from build123d import *

# Parameters (mm, degrees)
SKETCH1_W                = 38
SKETCH1_H                = 33
SKETCH1_R                = 1.7
BOSS_EXTRUDE1_DEPTH      = 3
BOSS_EXTRUDE2_DEPTH      = 5
BOSS_EXTRUDE2_DEPTH_BACK = 4
SKETCH3_R                = 0.75
SKETCH3_W                = 23.2
SKETCH3_H                = 12.2
FILLET1_R                = 2
CHAMFER1_SIZE            = 1.5
CHAMFER2_SIZE            = 3
CHAMFER2_SIZE_2          = 7


with BuildPart() as part:
    # Sketch1 → Boss-Extrude1 (new body)
    with BuildSketch(Plane.XY):
        Rectangle(SKETCH1_W, SKETCH1_H)
        with Locations((-13, 10.5)):
            Circle(SKETCH1_R, mode=Mode.SUBTRACT)
        with Locations((13, 10.5)):
            Circle(SKETCH1_R, mode=Mode.SUBTRACT)
        with Locations((13, -10.5)):
            Circle(SKETCH1_R, mode=Mode.SUBTRACT)
        with Locations((-13, -10.5)):
            Circle(SKETCH1_R, mode=Mode.SUBTRACT)
    extrude(amount=BOSS_EXTRUDE1_DEPTH)

    # Sketch3 → Boss-Extrude2 (add, two sides: drawn at the far end of the back side and taken through both)
    with BuildSketch(Plane(origin=(0, 0, 0), x_dir=(-1, 0, 0), z_dir=(0, -1, 0)).offset(-BOSS_EXTRUDE2_DEPTH_BACK)):
        Polygon((16.6, -3), (16.6, -16), (12.612805852, -20), (-12.612805852, -20), (-16.6, -16), (-16.6, -3), align=None)
        with Locations(Location((-13.85, -11.6, 0), (0, 0, 90))):
            Circle(SKETCH3_R, mode=Mode.SUBTRACT)
        with Locations(Location((13.85, -11.6, 0), (0, 0, 90))):
            Circle(SKETCH3_R, mode=Mode.SUBTRACT)
        with Locations((0, -11.6)):
            Rectangle(SKETCH3_W, SKETCH3_H, mode=Mode.SUBTRACT)
    extrude(amount=BOSS_EXTRUDE2_DEPTH + BOSS_EXTRUDE2_DEPTH_BACK)

    # Fillet1
    fillet1_edges = [part.edges().sort_by_distance(p)[0] for p in [
        (19, -16.5, 1.5),
        (-19, -16.5, 1.5),
        (-19, 16.5, 1.5),
        (19, 16.5, 1.5),
    ]]
    fillet(fillet1_edges, radius=FILLET1_R)

    # Chamfer1
    chamfer1_edges = [part.edges().sort_by_distance(p)[0] for p in [
        (-14.7, 10.5, 3),
        (11.3, 10.5, 3),
        (11.3, -10.5, 3),
        (-14.7, -10.5, 3),
    ]]
    chamfer(chamfer1_edges, length=CHAMFER1_SIZE)

    # Chamfer2
    # the kernel refuses this chamfer: 7, 3 mm, written as the material it takes off along each edge
    with BuildSketch(Plane(origin=(-11.6, -5, 17.7), x_dir=(-0.9965941369752023, -0.08246287738523173, 0), z_dir=(0, 0, -1))) as chamfer2_piece_1:
        Polygon((CHAMFER2_SIZE * 0.996594136975, CHAMFER2_SIZE * 0.0824628773852), (-CHAMFER2_SIZE_2 * 0.0824628773852, CHAMFER2_SIZE_2 * 0.996594136975), (0, 0), align=None)
    extrude(amount=12.2, mode=Mode.SUBTRACT)


solid = part.part
Part model, mm, in its own coordinate system. A direction names the side the tool comes from. Round coordinates to 2 decimals unless told otherwise and drop trailing zeros. Write each loop counter-clockwise with the first axis right and the second up, starting at its lowest first coordinate (ties: lowest second). Pieces come first, ordered by that corner, then holes. Notation, with made-up numbers: M 24,88.5 L 51,88.5 A25 cw 51,119.5 Z; hole C 43.5,-35 d9. An arc over 180 degrees is marked long. Return JSON: item names as keys, results as strings. Group by question number.
(1) Saw through at D-D on y = -2. Write the cut outline in (x, z), then the cut area to 3 significant figures.
(2) Saw through at B-B on z = 8.5. Write the cut outline in (x, y).
(3) Saw through at A-A on x = -1.5. Write the cut outline in (y, z).
(4) Which spindle directions (+Z, -Z, +X, -X, +Y, -Y) get a long thin tool onto all of the face, cutting with end or side? Do faces 1 (the face through (11.6, 0, 12)), 2 (the face through (2, -5, 5)), 3 (the face through (0, 0, 20)). Say none if no direction does.
(5) Drill centre lines: probe 1 along Y at (x, z) = (-13, 0.8); probe 2 along Z at (x, y) = (-5.5, 0.5); probe 3 along Y at (x, z) = (-12.5, 4.75). Where is each one in solid material? Low to high.
(6) Saw through at C-C on y = -10.5. Write the cut outline in (x, z), then the cut area to 3 significant figures.
(7) Pin check, flat tips, straight feed: pin 1 Ø0.6 at (y, z) = (3.5, 9.5) entering from +X; pin 2 Ø7 at (y, z) = (1, 11.5) entering from -X; pin 3 Ø2.5 at (x, y) = (13, 10.5) entering from +Z; pin 4 Ø6 at (x, y) = (-4, -12.5) entering from +Z. Stop position of each tip, or through.
(8) Two-plate mould, pull along X, no slides. Class faces 4 (the face through (0, 0, 0)), 5 (the face through (-11.6, 3, 12)), 6 (the face through (-19, 0, 1)): +X half, -X half, draft (parallel to the pull), parting line (faces both ways), or undercut.
Returned:
{
 "1": {"outline": "M -19,0 L 19,0 L 19,3 L 16.6,3 L 16.6,16 L 12.61,20 L -12.61,20 L -16.6,16 L -16.6,3 L -19,3 Z; hole M -13.31,5.5 L 11.6,5.5 L 11.6,17.7 L -13.31,17.7 L -13.31,12.12 A0.75 ccw long -13.31,11.08 Z; hole C 13.85,11.6 d1.5", "area": "355 mm²"},
 "2": {"outline": "M -16.6,-5 L -14.6,-5 L -11.6,2 L -11.6,4 L -16.6,4 Z; M 11.6,-5 L 16.6,-5 L 16.6,4 L 11.6,4 Z"},
 "3": {"outline": "M -16.5,0 L 16.5,0 L 16.5,3 L 4,3 L 4,5.5 L -5,5.5 L -5,3 L -16.5,3 Z; M -5,17.7 L 4,17.7 L 4,20 L -5,20 Z"},
 "4": {"face 1": "+Y, -Y", "face 2": "+Z, +X, -X, -Y", "face 3": "+Z, +X, -X, +Y, -Y"},
 "5": {"probe 1": "-16.5 to -12.2, -8.8 to 8.8, 12.2 to 16.5", "probe 2": "0 to 5.5, 17.7 to 20", "probe 3": "-5 to 4"},
 "6": {"outline": "M -19,0 L -14.7,0 L -14.7,1.5 L -16.2,3 L -19,3 Z; M -11.3,0 L 11.3,0 L 11.3,1.5 L 9.8,3 L -9.8,3 L -11.3,1.5 Z; M 14.7,0 L 19,0 L 19,3 L 16.2,3 L 14.7,1.5 Z", "area": "89.1 mm²"},
 "7": {"pin 1": "x = 16.6", "pin 2": "x = -16.6", "pin 3": "through", "pin 4": "z = 3"},
 "8": {"face 4": "draft", "face 5": "undercut", "face 6": "-X half"}
}
